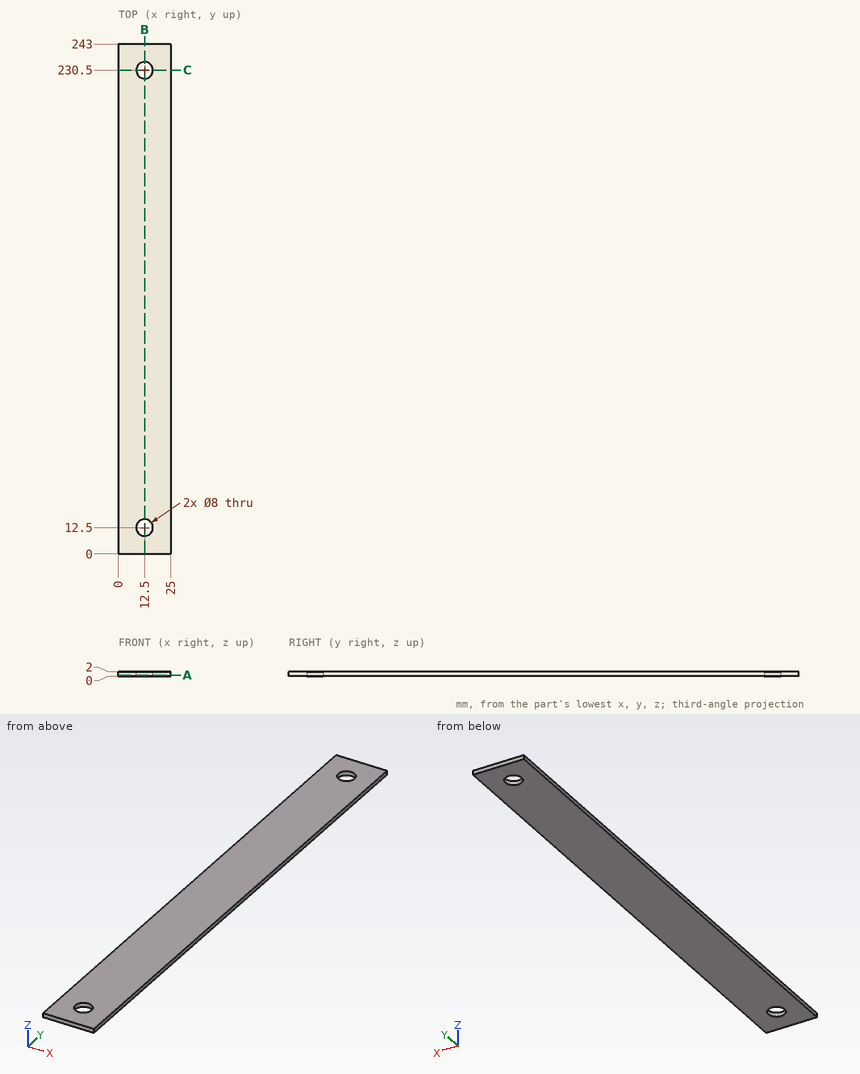
Geometry: see drawing. Coordinates: mm, zero at the bounding-box minimum. Round coordinates to 2 decimals unless told otherwise and drop trailing zeros. Loops run counter-clockwise (first coordinate to the right, second up) from the corner with the lowest first, then second, coordinate; pieces in that order, holes last. Notation, with made-up numbers: (16.5, -28) -> (23.5, -28) arc R20 ccw to (23.5, -8) -> close; hole circle Ø3 at (-3, 28). An arc over 180 degrees is marked (long way). Write each question's results on one line, items separated by ' | '.
Item 1: Cut plane A-A on z = 0.4. Return the cut outline in (x, y), and give its area (3 significant figures).
Answers below:
outline: (0, 0) -> (25, 0) -> (25, 243) -> (0, 243) -> close; hole circle Ø8 at (12.5, 12.5); hole circle Ø8 at (12.5, 230.5) | area: 5,970 mm²
Item 2: Cut plane C-C on y = 230.5. Return the cut outline in (x, z), and give its area (3 significant figures).
Answers below:
outline: (0, 0) -> (8.5, 0) -> (8.5, 2) -> (0, 2) -> close; (16.5, 0) -> (25, 0) -> (25, 2) -> (16.5, 2) -> close | area: 34.0 mm²
Item 3: Line query: probe 1 along Y at (x, z) = (12.5, 1.25); probe 2 along X at (y, z) = (12.5, 0.8); probe 3 along X at (y, z) = (15.5, 1.6). Output: solid intervals per line, ascending. Write a range as [from, to].
Answers below:
probe 1: y = [0, 8.5], [16.5, 226.5], [234.5, 243] | probe 2: x = [0, 8.5], [16.5, 25] | probe 3: x = [0, 9.85], [15.15, 25]
Item 4: Pin query (flat end, axial travel): pin 1 Ø1 at (x, y) = (7, 96.5) entering from -Z. Return the tip coordinate at first contact, or that it passes through.
Answers below:
pin 1: stops at z = 0
Item 5: Cut plane B-B on x = 12.5. Return the cut outline in (y, z), and give its area (3 significant figures).
Answers below:
outline: (0, 0) -> (8.5, 0) -> (8.5, 2) -> (0, 2) -> close; (16.5, 0) -> (226.5, 0) -> (226.5, 2) -> (16.5, 2) -> close; (234.5, 0) -> (243, 0) -> (243, 2) -> (234.5, 2) -> close | area: 454 mm²
